The drawing under review shows one solid part. Ordinate dimensions are in mm from its lowest x, y, z. A direction names the side the tool comes from. Coordinates: 2 decimals unless noted, no trailing zeros. Write each loop counter-clockwise with the first axis right and the second up, starting at its lowest first coordinate (ties: lowest second). Pieces come first, ordered by that corner, then holes.
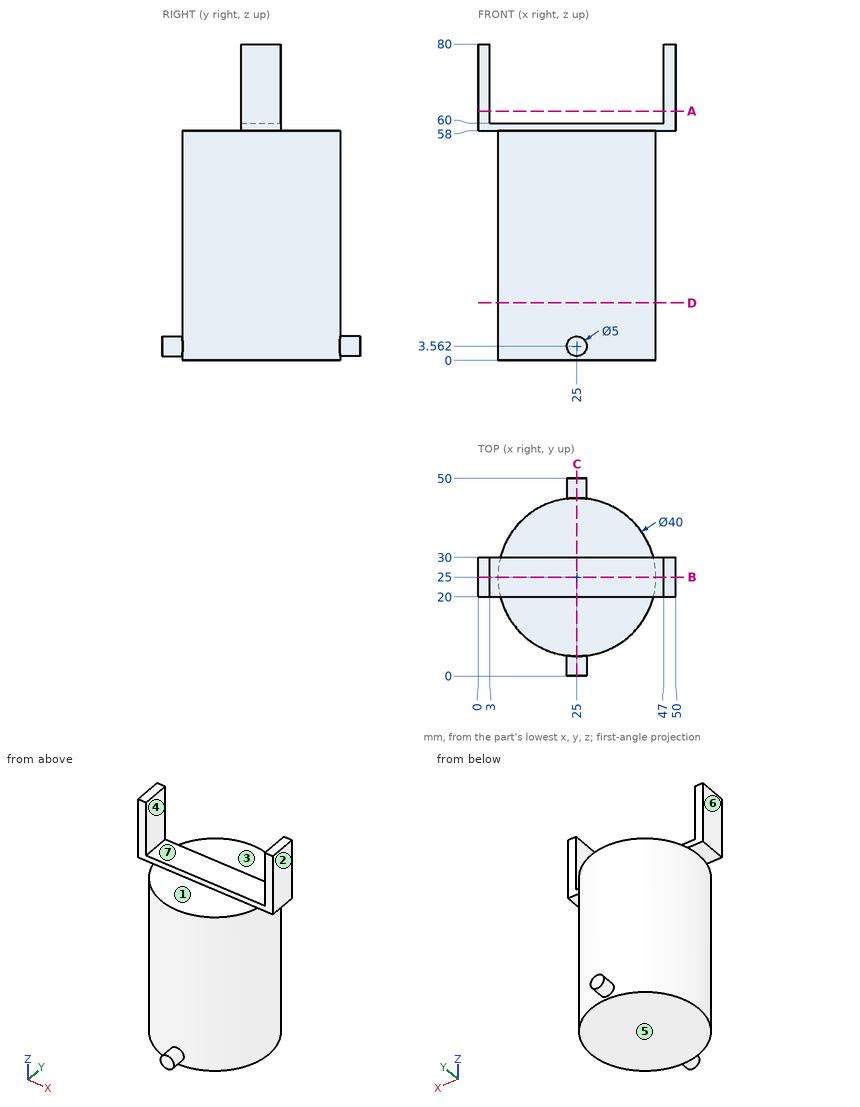
Q1. Draft analysis for pull direction X (two halves, no side actions). For the marked faces 4, 5, 6 and 7, state which applies: +X half, -X half, draft (parallel to the pull), parting line (faces both ways), or undercut.
Ans:
face 4: undercut
face 5: draft
face 6: -X half
face 7: undercut
Q2. Add section B-B (y = 25). State the section outline as (x, z) points.
Ans:
outline: (0, 58) - (5, 58) - (5, 0) - (45, 0) - (45, 58) - (50, 58) - (50, 80) - (47, 80) - (47, 60) - (3, 60) - (3, 80) - (0, 80) - close
Q3. Add section D-D (z = 14.5). State the section outline as (x, y) points.
Ans:
outline: circle Ø40 at (25, 25)
Q4. Clearance check with flat-ended pins moving along their axes: pin 1 Ø3 at (y, z) = (26.5, 44) entering from -X; pin 2 Ø5 at (x, y) = (29, 33) entering from +Z; pin 3 Ø12 at (y, z) = (42.5, 47.5) entering from -X. State where each tip first meets the part, or that it passes through.
Ans:
pin 1: stops at x = 5
pin 2: stops at z = 58
pin 3: stops at x = 8.64
Q5. Add section A-A (z = 63). State the section outline as (x, y) points, then the cut area to 3 significant figures.
Ans:
outline: (0, 20) - (3, 20) - (3, 30) - (0, 30) - close; (47, 20) - (50, 20) - (50, 30) - (47, 30) - close
area: 60.0 mm2
Q6. For probe 1 along X at (y, z) = (24.5, 15.5); probe 2 along X at (y, z) = (30, 12.5) (1 decimal); probe 3 along Z at (x, y) = (13.5, 17), list the stretches that pass through material, from the lowest coordinate up.
Ans:
probe 1: x = 5.01 to 44.99
probe 2: x = 5.6 to 44.4
probe 3: z = 0 to 58
Q7. Add section C-C (x = 25). State the section outline as (y, z) points, then the cut area to 3 significant figures.
Ans:
outline: (0, 1.06) - (5, 1.06) - (5, 0) - (45, 0) - (45, 1.06) - (50, 1.06) - (50, 6.06) - (45, 6.06) - (45, 58) - (30, 58) - (30, 60) - (20, 60) - (20, 58) - (5, 58) - (5, 6.06) - (0, 6.06) - close
area: 2,390 mm2
Q8. Tool access review of the marked faces 1, 2 and 3: name each direction out of +Z, -Z, +X, -X, +Y, -Y from which nothing blocks a thin tool from reaching the whole face with its end or side.
Ans:
face 1: +Z, +X, -X, -Y
face 2: +Z, -Z, +X, +Y, -Y
face 3: +Z, +X, -X, +Y
